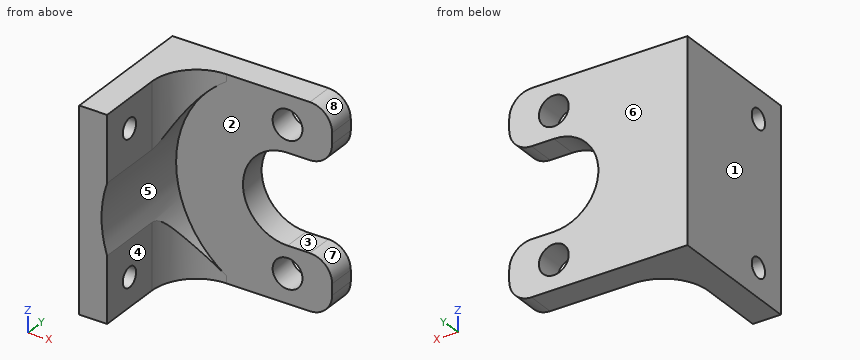
from build123d import *

# Parameters (mm, degrees)
SKETCH1_W             = 20.32
SKETCH1_H             = 22.86
BOSS_EXTRUDE1_DEPTH   = 3.175
FILLET1_R             = 2.54
FILLET2_R             = 2.54
CUT_EXTRUDE2_DEPTH    = 4.175
FILLET3_R             = 2.54
FILLET4_R             = 2.54
SKETCH4_W             = 3.175
SKETCH4_H             = 22.86
BOSS_EXTRUDE2_DEPTH   = 12.7
FILLET6_R             = 5.08
SKETCH5_R             = 12.7
CUT_EXTRUDE4_DEPTH    = 13.7
F_4_40_TAPPED_HOLE3_D = 2.2606
M3_CLEARANCE_HOLE1_D  = 3.4


with BuildPart() as part:
    # Sketch1 → Boss-Extrude1 (new body)
    with BuildSketch(Plane(origin=(0, 0, 0), x_dir=(1, 0, 0), z_dir=(0, 1, 0))):
        Rectangle(SKETCH1_W, SKETCH1_H)
    extrude(amount=BOSS_EXTRUDE1_DEPTH)

    # Fillet1
    fillet1_edges = [part.edges().sort_by_distance(p)[0] for p in [
        (10.16, 1.5875, -11.43),
    ]]
    fillet(fillet1_edges, radius=FILLET1_R)

    # Fillet2
    fillet2_edges = [part.edges().sort_by_distance(p)[0] for p in [
        (10.16, 1.5875, 11.43),
    ]]
    fillet(fillet2_edges, radius=FILLET2_R)

    # Sketch2 → Cut-Extrude2 (cut, through all)
    with BuildSketch(Plane.XZ):
        with BuildLine():
            Line((5.08, -5.08), (10.16, -5.08))
            Line((10.16, -5.08), (10.16, 5.08))
            Line((10.16, 5.08), (5.08, 5.08))
            ThreePointArc((5.08, 5.08), (0, 0), (5.08, -5.08))
        make_face()
    extrude(amount=-CUT_EXTRUDE2_DEPTH, mode=Mode.SUBTRACT)

    # Fillet3
    fillet3_edges = [part.edges().sort_by_distance(p)[0] for p in [
        (10.16, 1.5875, 5.08),
    ]]
    fillet(fillet3_edges, radius=FILLET3_R)

    # Fillet4
    fillet4_edges = [part.edges().sort_by_distance(p)[0] for p in [
        (10.16, 1.5875, -5.08),
    ]]
    fillet(fillet4_edges, radius=FILLET4_R)

    # Sketch4 → Boss-Extrude2 (add)
    with BuildSketch(Plane.XZ):
        with Locations((-8.5725, 0)):
            Rectangle(SKETCH4_W, SKETCH4_H)
    extrude(amount=BOSS_EXTRUDE2_DEPTH)

    # Fillet6
    fillet6_edges = [part.edges().sort_by_distance(p)[0] for p in [
        (-6.985, 0, 0),
    ]]
    fillet(fillet6_edges, radius=FILLET6_R)

    # Sketch5 → Cut-Extrude4 (cut, through all)
    with BuildSketch(Plane.XZ):
        with Locations((5.08, 0)):
            Circle(SKETCH5_R)
    extrude(amount=CUT_EXTRUDE4_DEPTH, mode=Mode.SUBTRACT)

    # #4-40 Tapped Hole3 (through all)
    with Locations(Plane(origin=(-6.985, 0, 0), x_dir=(0, 0, -1), z_dir=(1, 0, 0))):
        with Locations((-8.128, -8.89), (8.128, -8.89)):
            Hole(F_4_40_TAPPED_HOLE3_D / 2)

    # M3 Clearance Hole1 (through all)
    with Locations(Plane(origin=(0, 0, 0), x_dir=(-1, 0, 0), z_dir=(0, -1, 0))):
        with Locations((-5.08, -8.128), (-5.08, 8.128)):
            Hole(M3_CLEARANCE_HOLE1_D / 2)


solid = part.part
The listing builds one solid part. Answer for the finished solid, in the listing's coordinates (mm). Face numbers are marked on the shaded views. A direction names the side the tool comes from. Give positions to 0.01 mm unless a question says otherwise; leave off trailing zeros. Write each loop counter-clockwise with the first axis right and the second up, starting at its lowest first coordinate (ties: lowest second). Pieces come first, ordered by that corner, then holes.
Item 1: Determine the mould class of the marked faces 5, 6, 7 and 8 for opening direction Z: released by +Z, released by -Z, zero draft, split by the parting line, or undercut.
Item 2: Find the intervals of material crossed by line 1 along Z through (x, y) = (5.08, 2.1); line 2 along Y through (x, z) = (-9, -8) (3 decimals); line 3 along Z through (x, y) = (-9.5, -9.25), in increasing order.
Item 3: Section A-A, the plane y = -8.89 is taken. Write down the section's boundary in (x, z) (3 decimals), plus the area to 3 significant figures.
Item 4: Which of the six approach directions +Z, -Z, +X, -X, +Y, -Y give full straight-line access (tool end or side, diameter ignored) to the marked faces 1, 2, 3 and 4?
Item 5: Flat-ended cylindrical pins translate along their axes: P1, Ø8, axis at y = -8, z = 7, coming from the +X side; P2, Ø6, axis at y = -9.5, z = -8.5, coming from the +X side (3 decimals); P3, Ø6, axis at x = 4.5, y = -5.5, coming from the +Z side; P4, Ø5.5, axis at x = 0.5, z = -4.5, coming from the -Y side. Find the tip coordinate at first contact, or state that the pin passes through.
Item 6: Section B-B, the plane x = 4.75 is taken. Write down the section's boundary in (y, z) (3 decimals), plus the area to 3 significant figures.
Item 7: Section D-D, the plane z = 0 is taken. Write down the section's boundary in (x, y) (3 decimals), plus the area to 3 significant figures.
Item 8: Section C-C, the plane y = -5.75 is taken. Write down the section's boundary in (x, z) (3 decimals), plus the area to 3 significant figures.
Completed:
1. face 5: undercut
1. face 6: zero draft
1. face 7: undercut
1. face 8: released by +Z
2. line 1: z = -11.43 to -9.83, -6.43 to -5.08, 5.08 to 6.43, 9.83 to 11.43
2. line 2: y = -12.7 to -10.013, -7.767 to 3.175
2. line 3: z = -11.43 to -9.2, -7.06 to 7.06, 9.2 to 11.43
3. outline: (-10.16, -11.43) - (-6.985, -11.43) - (-6.985, -9.258) - (-10.16, -9.258) - close; (-10.16, -6.998) - (-6.985, -6.998) - (-6.985, -3.966) arc R12.7 cw to (-6.985, 3.966) - (-6.985, 6.998) - (-10.16, 6.998) - close; (-10.16, 9.258) - (-6.985, 9.258) - (-6.985, 11.43) - (-10.16, 11.43) - close
3. area: 54.9 mm2
4. face 1: +Z, -Z, -X, +Y, -Y
4. face 2: +X, -Y
4. face 3: +X, +Y, -Y
4. face 4: +Z, -Z, +X, -Y
5. P1: stops at x = -6.87
5. P2: stops at x = -6.985
5. P3: passes through
5. P4: stops at y = 0
6. outline: (0, -11.43) - (3.175, -11.43) - (3.175, -9.796) - (0, -9.796) - close; (0, -6.46) - (3.175, -6.46) - (3.175, -5.069) - (0, -5.069) - close; (0, 5.069) - (3.175, 5.069) - (3.175, 6.46) - (0, 6.46) - close; (0, 9.796) - (3.175, 9.796) - (3.175, 11.43) - (0, 11.43) - close
6. area: 19.2 mm2
7. outline: (-10.16, -12.7) - (-7.62, -12.7) - (-7.62, 0) - (0, 0) - (0, 3.175) - (-10.16, 3.175) - close
7. area: 64.5 mm2
8. outline: (-10.16, -11.43) - (-6.985, -11.43) - (-6.985, -3.966) arc R12.7 cw to (-6.985, 3.966) - (-6.985, 11.43) - (-10.16, 11.43) - close
8. area: 69.2 mm2
